The drawing under review shows one solid part. Ordinate dimensions are in mm from its lowest x, y, z. A direction names the side the tool comes from. Coordinates: 2 decimals unless noted, no trailing zeros. Order: outer loops, then holes, each group sorted by start corner. A loop starts at its lowest first (then second) coordinate and runs counter-clockwise, first axis right, second up. Notation, with made-up numbers: (58, 78.25) -> (91, 78.25) arc R6 ccw to (91, 88.25) -> close; hole circle Ø4 at (39, -38). An arc over 180 degrees is marked (long way). Use a Markdown table: item, result. Add a question column.
Q1. Add section C-C (x = 97). State the section outline as (y, z) points.
Q2. Machinability: for the marked faces 1, 2 and 3, which of the approach directions +Z, -Z, +X, -X, +Y, -Y give a long, thin tool a straight path to every point of the face, cutting with its end or side? Answer none if there is none.
Q3. Add section A-A (y = 16.25). State the section outline as (x, z) points.
Q4. Insertion check: pin 1 (12.5 mm diameter, centred on x = 34, y = 11.5, fed in from +Z); pin 2 (7.5 mm diameter, centred on x = 91.5, y = 13, fed in from -Z). Each pin has a flat end and moves straight along its axis. Give the tip position at first contact, or say it passes through.
Q5. Add section B-B (z = 47). State the section outline as (x, y) points, then the cut area to 3 significant figures.
Q6. The part is to be moulded in two halves that separate along Z. For the marked faces 4, 5, 6 and 7, say which applies: pulls with the +Z half, pulls with the -Z half, needs draft (parallel to the pull), parting line crosses it, or undercut.
Q7. Wall thickness on probe 1 along X at (y, z) = (24, 76.5); probe 2 along Z at (x, y) = (61, 14.5); probe 3 along X at (y, z) = (18.5, 37): over which ranges is each line inside the solid? List them lowest first.
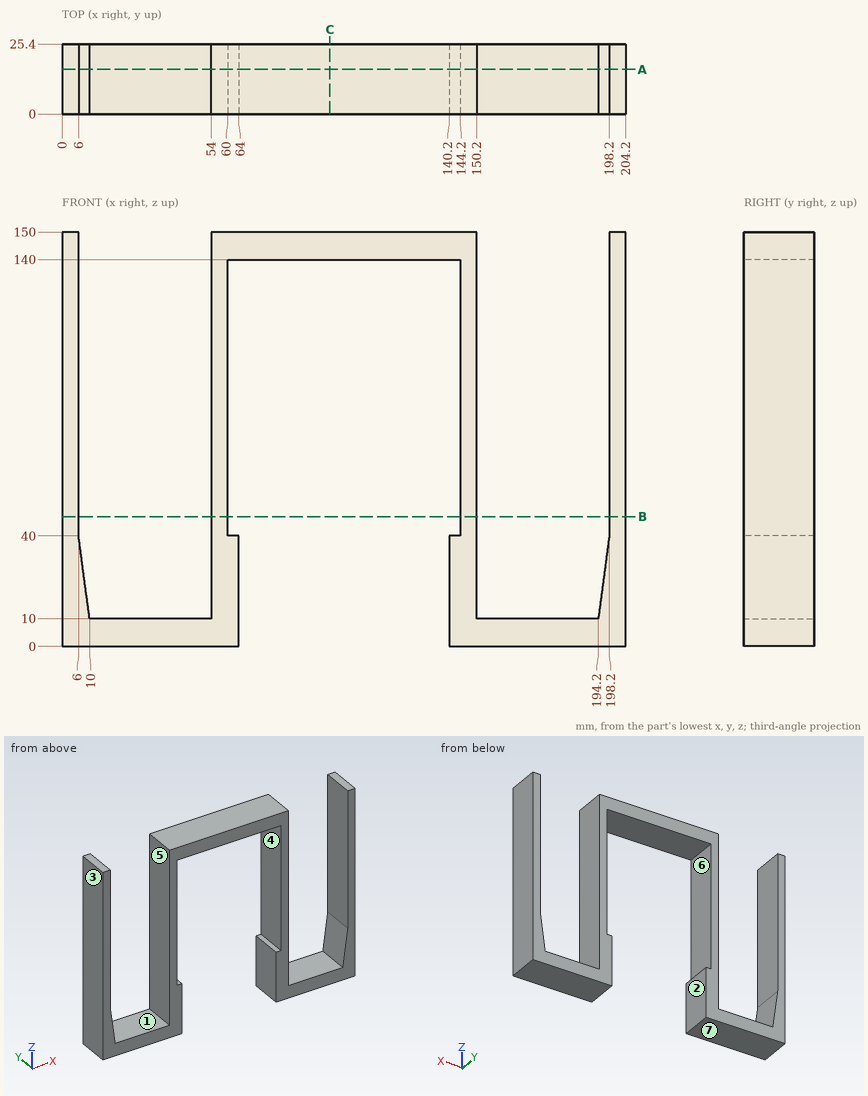
Established:
| question | item | result |
|---|---|---|
| 1 | outline | (0, 140) -> (25.4, 140) -> (25.4, 150) -> (0, 150) -> close |
| 2 | face 1 | +Z, +Y, -Y |
| 2 | face 2 | -Z, +Y, -Y |
| 2 | face 3 | +Z, -Z, -X, +Y, -Y |
| 3 | outline | (0, 0) -> (64, 0) -> (64, 40) -> (60, 40) -> (60, 140) -> (144.2, 140) -> (144.2, 40) -> (140.2, 40) -> (140.2, 0) -> (204.2, 0) -> (204.2, 150) -> (198.2, 150) -> (198.2, 40) -> (194.2, 10) -> (150.2, 10) -> (150.2, 150) -> (54, 150) -> (54, 10) -> (10, 10) -> (6, 40) -> (6, 150) -> (0, 150) -> close |
| 4 | pin 1 | z = 10 |
| 4 | pin 2 | z = 140 |
| 5 | outline | (0, 0) -> (6, 0) -> (6, 25.4) -> (0, 25.4) -> close; (54, 0) -> (60, 0) -> (60, 25.4) -> (54, 25.4) -> close; (144.2, 0) -> (150.2, 0) -> (150.2, 25.4) -> (144.2, 25.4) -> close; (198.2, 0) -> (204.2, 0) -> (204.2, 25.4) -> (198.2, 25.4) -> close |
| 5 | area | 610 mm^2 |
| 6 | face 4 | undercut |
| 6 | face 5 | needs draft |
| 6 | face 6 | undercut |
| 6 | face 7 | pulls with the -Z half |
| 7 | probe 1 | 0 to 6, 54 to 60, 144.2 to 150.2, 198.2 to 204.2 |
| 7 | probe 2 | 0 to 40, 140 to 150 |
| 7 | probe 3 | 0 to 6.4, 54 to 64, 140.2 to 150.2, 197.8 to 204.2 |
